```python
from build123d import *

# Parameters (mm, degrees)
F0_R     = 9.5
F1_DEPTH = 14.5
F2_R     = 3.15
F3_DEPTH = 13
F5_DEPTH = 12.5
F6_SIZE  = 4.49999
F7_W     = 1.4
F7_H     = 9.2790693743
F8_DEPTH = 0.3


# Not quite as in the source:
# - a fillet or chamfer is up to 0.001 mm smaller than in the source, because OpenCascade refuses the exact size


with BuildPart() as f1:
    # F0 (on Top) → F1 (new body)
    with BuildSketch(Plane.XY):
        Circle(F0_R)
    extrude(amount=F1_DEPTH)

    # F2 (on face) → F3 (cut)
    with BuildSketch(Plane(origin=(0, 0, 0), x_dir=(1, 0, 0), z_dir=(0, 0, -1))):
        Circle(F2_R)
    extrude(amount=-F3_DEPTH, mode=Mode.SUBTRACT)

    # F4 (on Front) → F5 (cut, symmetric)
    with BuildSketch(Plane.XZ):
        Polygon((5.0005883317, 16.3299063618), (3.68460026, 14.5), (5, 6.9363636364), (9.7186830602, 6.9363636364), (12.480460446, 14.9852110131), align=None)
        Polygon((-5, 6.9363636364), (-3.68460026, 14.5), (-5.0005883317, 16.3299063618), (-12.480460446, 14.9852110131), (-9.7186830602, 6.9363636364), align=None)
    extrude(amount=F5_DEPTH, both=True, mode=Mode.SUBTRACT)

    # F6 (size 4.5 in the source; OpenCascade refuses exactly that, so slightly less here)
    f6_edges = [f1.edges().sort_by_distance(p)[0] for p in [
        (8.299096, -4.623311, 6.936364),
        (8.299096, 4.623311, 6.936364),
        (-9.5, 0, 6.936364),
    ]]
    chamfer(f6_edges, length=F6_SIZE)

    # F7 (on face) → F8 (cut)
    with BuildSketch(Plane.XY.offset(14.5)):
        with Locations((0, -5.2029067301)):
            Rectangle(F7_W, F7_H)
    extrude(amount=-F8_DEPTH, mode=Mode.SUBTRACT)


solid = f1.part
```
The listing builds one solid part. Answer for the finished solid, in the listing's coordinates (mm). A direction names the side the tool comes from. Coordinates: 2 decimals unless noted, no trailing zeros. Loops run counter-clockwise (first coordinate to the right, second up) from the corner with the lowest first, then second, coordinate; pieces in that order, holes last. Notation, with made-up numbers: M -12,40 L 23,40 A13 ccw 23,51 Z; hole C 11.5,1.25 d3. An arc over 180 degrees is marked long. Answer as a JSON object with one key per item and string values. Group by question number.
Item 1: Determine the mould class of faces 1 (the face through (0, 0, 13)), 2 (the face through (-4.515, -0.123, 9.724)), 3 (the face through (4.486, 0.123, 9.893)) for opening direction X: +X half, -X half, draft (parallel to the pull), parting line (faces both ways), or undercut.
Item 2: Section B-B (x = 0) is taken. Write down the section's boundary in (y, z), and give its area (3 significant figures).
Item 3: Section C-C (z = 9.5) is taken. Write down the section's boundary in (x, y).
Item 4: Which of the six approach directions +Z, -Z, +X, -X, +Y, -Y give full straight-line access (tool end or side, diameter ignored) to faces 4 (the face through (-2.5, 1.917, 6.409)), 5 (the face through (0, -5, 14.2)), 6 (the face through (0, 0, 14.5))?
Item 5: Consider L1, parallel to Y at x = 0, z = 9; L2, parallel to X at y = 0, z = 5.25; L3, parallel to X at y = 0, z = 6.5. Determine where each line is inside the solid, lowest interval first.
Item 6: Each of these flat-tipped pins is pushed along its axis until it touches: P1, Ø1.5, axis at y = -1.5, z = 8.5, coming from the +X side; P2, Ø3, axis at x = -0.5, y = -0.5, coming from the -Z side; P3, Ø4, axis at y = -3, z = 6, coming from the -X side. Where does it stop, or does it pass through?
Item 7: Section A-A (z = 4) is taken. Write down the section's boundary in (x, y).
Item 8: Section D-D (x = 4) is taken. Write down the section's boundary in (y, z).
Solved:
{
 "1": {"face 1": "undercut", "face 2": "-X half", "face 3": "+X half"},
 "2": {"outline": "M -9.5,0 L -3.15,0 L -3.15,13 L 3.15,13 L 3.15,0 L 9.5,0 L 9.5,14.5 L -0.56,14.5 L -0.56,14.2 L -9.5,14.2 Z", "area": "191 mm2"},
 "3": {"outline": "M -4.55,-8.34 A9.5 ccw 4.55,-8.34 L 4.55,8.34 A9.5 ccw -4.55,8.34 Z; hole C 0,0 d6.3"},
 "4": {"face 4": "-Z", "face 5": "+Z, -Y", "face 6": "+Z, +X, -X, +Y, -Y"},
 "5": {"L1": "y = -9.5 to -3.15, 3.15 to 9.5", "L2": "x = -6.69 to -3.15, 3.15 to 6.69", "L3": "x = -5.44 to -3.15, 3.15 to 5.44"},
 "6": {"P1": "stops at x = 4.86", "P2": "stops at z = 13", "P3": "stops at x = -7.47"},
 "7": {"outline": "M -5.51,-7.74 A9.5 ccw 5.51,-7.74 L 5.51,-5.71 A7.94 ccw 5.51,5.71 L 5.51,7.74 A9.5 ccw -5.51,7.74 L -5.51,5.71 A7.94 ccw -5.51,-5.71 Z; hole C 0,0 d6.3"},
 "8": {"outline": "M -8.62,0 L 8.62,0 L 8.62,12.69 L -8.62,12.69 Z"}
}
